Could you check a few things on this model? Use its own coordinates, in mm. A direction names the side the tool comes from. Coordinates: 2 decimals unless noted, no trailing zeros. Loops run counter-clockwise (first coordinate to the right, second up) from the corner with the lowest first, then second, coordinate; pieces in that order, holes last. Notation, with made-up numbers: M 77.25,33.25 L 128.25,33.25 A25 ccw 128.25,46.25 Z; hole C 61.25,55.5 d11. An arc over 180 degrees is marked long. Return JSON: item names as keys, results as strings. Group by question number.
from build123d import *

# Parameters (mm, degrees)
SKETCH4_R           = 3
BOSS_EXTRUDE1_DEPTH = 2
SKETCH9_R           = 1.5
CUT_EXTRUDE1_DEPTH  = 6
SKETCH10_R          = 2
CUT_EXTRUDE2_DEPTH  = 0.5


with BuildPart() as part:
    # Sketch2 → Revolve6 (revolve)
    with BuildSketch(Plane(origin=(0, 0, 0), x_dir=(0, 0, -1), z_dir=(1, 0, 0))):
        with BuildLine():
            Line((26.5077562, 274.996982717), (26.5077562, 273.848618937))
            Line((26.5077562, 273.848618937), (39.220771912, 273.848618937))
            Line((39.220771912, 273.848618937), (46.181267187, 321.561079724))
            Line((46.181267187, 321.561079724), (44.775299462, 321.561079724))
            Line((44.775299462, 321.561079724), (40.547674755, 314.238618937))
            Line((40.547674755, 314.238618937), (40.547674755, 295.540718438))
            add(Edge.make_bspline(
                [(40.547674755, 295.540718438), (40.447740466, 295.012709616), (40.292777353, 293.970757619), (39.930889755, 292.587532753), (39.516186416, 291.581451359), (39.108370782, 290.57804728), (38.439698054, 289.316986818), (37.331416086, 288.032583079), (36.368363881, 287.115418474), (35.630231264, 286.340079673), (35.016472726, 285.762737126), (34.394259795, 285.247169223), (33.635524662, 284.556557999), (32.920361334, 283.771384038), (32.129651901, 282.986073936), (31.485241784, 282.459482323), (30.914997208, 281.963476573), (30.371700346, 281.391298159), (29.782796159, 280.80462685), (29.227584581, 280.262154528), (28.724752618, 279.674853681), (28.180386253, 279.039651715), (27.651838315, 278.470209992), (27.308145935, 277.876839187), (26.995230081, 277.127164256), (26.597952618, 276.164510632), (26.464811583, 275.470548141), (26.5077562, 274.996982717)],
                knots=[0, 0, 0, 0, 0.062544048, 0.125088096, 0.156360121, 0.187632145, 0.250176193, 0.312720241, 0.375264289, 0.406536313, 0.437808337, 0.469080362, 0.500352386, 0.562896434, 0.594168458, 0.625440482, 0.656712506, 0.68798453, 0.719256554, 0.750528579, 0.781800603, 0.813072627, 0.844344651, 0.875616675, 0.906888699, 0.938160723, 1.000704771, 1.000704771, 1.000704771, 1.000704771], degree=3))
        make_face()
    revolve(axis=Axis((0, 5, 0), (0, 1, 0)))

    # Sketch4 → Boss-Extrude1 (add)
    with BuildSketch(Plane.XZ.offset(-273.848618937)):
        with Locations(Location((-31.176914536, 18, 0), (0, 0, 270))):
            Circle(SKETCH4_R)
        with Locations(Location((36, 0, 0), (0, 0, 270))):
            Circle(SKETCH4_R)
    extrude(amount=BOSS_EXTRUDE1_DEPTH)

    # Sketch9 → Cut-Extrude1 (cut)
    with BuildSketch(Plane.XZ.offset(-271.848618937)):
        with Locations(Location((36, 0, 0), (0, 0, 270))):
            Circle(SKETCH9_R)
        with Locations(Location((-31.176914536, 18, 0), (0, 0, 270))):
            Circle(SKETCH9_R)
    extrude(amount=-CUT_EXTRUDE1_DEPTH, mode=Mode.SUBTRACT)

    # Sketch10 → Cut-Extrude2 (cut)
    with BuildSketch(Plane.XZ.offset(-271.848618937)):
        with Locations(Location((36, 0, 0), (0, 0, 270))):
            Circle(SKETCH10_R)
        with Locations(Location((-31.176914536, 18, 0), (0, 0, 270))):
            Circle(SKETCH10_R)
    extrude(amount=-CUT_EXTRUDE2_DEPTH, mode=Mode.SUBTRACT)

    # Chamfer3: read off the stored shape, not the designer's step
    # Chamfer3: loft between two sections, ruled curve by curve
    chamfer3_from = [
        Edge.make_three_point_arc((-31.176914536, 272.348618937, 15.95), (-29.126914536, 272.348618937, 18), (-31.176914536, 272.348618937, 20.05)),
        Edge.make_three_point_arc((-31.176914536, 272.348618937, 20.05), (-33.226914536, 272.348618937, 18), (-31.176914536, 272.348618937, 15.95)),
    ]
    chamfer3_to = [
        Edge.make_three_point_arc((-31.176914536, 271.848618937, 15.45), (-28.626914536, 271.848618937, 18), (-31.176914536, 271.848618937, 20.55)),
        Edge.make_three_point_arc((-31.176914536, 271.848618937, 20.55), (-33.726914536, 271.848618937, 18), (-31.176914536, 271.848618937, 15.45)),
    ]
    chamfer3 = Solid(Shell([*[Face.make_surface_from_curves(chamfer3_from[k], chamfer3_to[k]) for k in range(2)], Face(Wire(chamfer3_from)), Face(Wire(chamfer3_to))]))
    add(chamfer3, mode=Mode.SUBTRACT)

    # Chamfer3 2: loft between two sections, ruled curve by curve
    chamfer3_2_from = [
        Edge.make_three_point_arc((36, 272.348618937, -2.05), (38.05, 272.348618937, 0), (36, 272.348618937, 2.05)),
        Edge.make_three_point_arc((36, 272.348618937, 2.05), (33.95, 272.348618937, 0), (36, 272.348618937, -2.05)),
    ]
    chamfer3_2_to = [
        Edge.make_three_point_arc((36, 271.848618937, -2.55), (38.55, 271.848618937, 0), (36, 271.848618937, 2.55)),
        Edge.make_three_point_arc((36, 271.848618937, 2.55), (33.45, 271.848618937, 0), (36, 271.848618937, -2.55)),
    ]
    chamfer3_2 = Solid(Shell([*[Face.make_surface_from_curves(chamfer3_2_from[k], chamfer3_2_to[k]) for k in range(2)], Face(Wire(chamfer3_2_from)), Face(Wire(chamfer3_2_to))]))
    add(chamfer3_2, mode=Mode.SUBTRACT)


solid = part.part
(1) Will these pins go through, and if not, where does the flat tip stop? P1, Ø10, axis at y = 286.5, z = 3, coming from the -X side; P2, Ø1, axis at x = -2.5, z = -36.5, coming from the +Y side; P3, Ø2.5, axis at x = -31.18, z = 18, coming from the +Y side.
(2) For faces 4 (the face through (39.583, 304.759, 8.79)), 5 (the face through (-32.09, 275.06, 19.19)), 6 (the face through (25.877, 274.415, 5.746)), which set-ups out of +Z, -Z, +X, -X, +Y, -Y let a thin tool reach every point of the face, with its end or its side?
(3) We'd pull the mould along X, two halves only. Please class faces 1 (the face through (-29.15, 272.86, 20.21)), 2 (the face through (-33, 272.349, 18)), 3 (the face through (38, 271.849, 2)): +X half, -X half, draft (parallel to the pull), parting line (faces both ways), or undercut.
(4) Imagine slicing it at A-A, the plane y = 306.5. Write out the boundary of the cut face in (x, z).
(5) If I drill on L1, parallel to X at y = 274.6, z = 0; L2, parallel to X at y = 273.7, z = 18; L3, parallel to X at y = 318.5, z = -30, over which ranges is the centre line in solid material (lowest first)? Write a range as [from, to].
Checks:
{
 "1": {"P1": "x = -41.74", "P2": "y = 287.82", "P3": "y = 287.99"},
 "2": {"face 4": "+Y", "face 5": "-Y", "face 6": "+Y, -Y"},
 "3": {"face 1": "parting line", "face 2": "undercut", "face 3": "draft"},
 "4": {"outline": "C 0,0 d87.97; hole C 0,0 d81.1"},
 "5": {"L1": "[-39.33, -26.51], [26.51, 34.5], [37.5, 39.33]", "L2": "[-34.18, -32.68], [-29.68, -28.18]", "L3": "[-34.52, -30.82], [30.82, 34.52]"}
}
